from build123d import *

# Parameters (mm, degrees)
PAD_DEPTH       = 3.2
PAD001_DEPTH    = 15.2
POCKET_DEPTH    = 16.6
SKETCH003_R     = 4.1
SKETCH003_R_2   = 1
SKETCH003_R_3   = 3.2
POCKET001_DEPTH = 1.8
SKETCH004_W     = 26.8
SKETCH004_H     = 1.6
PAD002_DEPTH    = 5
CHAMFER_SIZE    = 1.2
POCKET002_DEPTH = 1
SKETCH006_R     = 4.5
SKETCH006_R_2   = 1.7
PAD003_DEPTH    = 3.4
CHAMFER001_SIZE = 0.4
SKETCH007_R     = 1.7
POCKET003_DEPTH = 21.801
SKETCH008_R     = 2.7
POCKET004_DEPTH = 0.6
CHAMFER002_SIZE = 0.8
SKETCH009_R     = 4
POCKET005_DEPTH = 1
SKETCH010_R     = 3
SKETCH010_R_2   = 1.2
PAD004_DEPTH    = 1.6
CHAMFER003_SIZE = 0.4
CHAMFER004_SIZE = 0.8


with BuildPart() as part:
    # Sketch → Pad (new body)
    with BuildSketch(Plane.XY):
        with BuildLine():
            Line((-21, 45), (21, 45))
            ThreePointArc((25, 41), (23.828427, 43.828427), (21, 45))
            Line((25, 41), (25, -41))
            ThreePointArc((21, -45), (23.828427, -43.828427), (25, -41))
            Line((21, -45), (-21, -45))
            ThreePointArc((-25, -41), (-23.828427, -43.828427), (-21, -45))
            Line((-25, -41), (-25, 41))
            ThreePointArc((-21, 45), (-23.828427, 43.828427), (-25, 41))
        make_face()
    extrude(amount=PAD_DEPTH)

    # Sketch001 (on Face9 of Pad) → Pad001 (join)
    with BuildSketch(Plane(origin=(0, 0, 0), x_dir=(1, 0, 0), z_dir=(0, 0, -1))):
        with BuildLine():
            Line((-12, 35), (12, 35))
            ThreePointArc((15, 32), (14.12132, 34.12132), (12, 35))
            Line((15, 32), (15, -32))
            ThreePointArc((12, -35), (14.12132, -34.12132), (15, -32))
            Line((12, -35), (-12, -35))
            ThreePointArc((-15, -32), (-14.12132, -34.12132), (-12, -35))
            Line((-15, -32), (-15, 32))
            ThreePointArc((-12, 35), (-14.12132, 34.12132), (-15, 32))
        make_face()
    extrude(amount=PAD001_DEPTH)

    # Sketch002 (on Face5 of Pad001) → Pocket (cut)
    with BuildSketch(Plane.XY.offset(3.2)):
        with BuildLine():
            Line((-11.2, 33.4), (11.2, 33.4))
            ThreePointArc((13.4, 31.2), (12.755635, 32.755635), (11.2, 33.4))
            Line((13.4, 31.2), (13.4, -31.2))
            ThreePointArc((11.2, -33.4), (12.755635, -32.755635), (13.4, -31.2))
            Line((11.2, -33.4), (-11.2, -33.4))
            ThreePointArc((-13.4, -31.2), (-12.755635, -32.755635), (-11.2, -33.4))
            Line((-13.4, -31.2), (-13.4, 31.2))
            ThreePointArc((-11.2, 33.4), (-12.755635, 32.755635), (-13.4, 31.2))
        make_face()
    extrude(amount=-POCKET_DEPTH, mode=Mode.SUBTRACT)

    # Sketch003 (on Face28 of Pocket) → Pocket001 (cut)
    with BuildSketch(Plane.XY.offset(-13.4)):
        with Locations((0, -24)):
            Circle(SKETCH003_R)
        with Locations((0, -10)):
            Circle(SKETCH003_R_2)
        with Locations((0, 10)):
            Circle(SKETCH003_R_3)
        with Locations((0, 25)):
            Circle(SKETCH003_R_2)
    extrude(amount=-POCKET001_DEPTH, mode=Mode.SUBTRACT)

    # Sketch004 (on Face28 of Pocket001) → Pad002 (join)
    with BuildSketch(Plane.XY.offset(-13.4)):
        Rectangle(SKETCH004_W, SKETCH004_H)
    extrude(amount=PAD002_DEPTH)

    # Chamfer
    chamfer_edges = [part.edges().sort_by_distance(p)[0] for p in [
        (-23.828427, 43.828427, 3.2),
        (-25, 0, 3.2),
        (0, 45, 3.2),
        (23.828427, 43.828427, 3.2),
        (25, 0, 3.2),
        (-23.828427, -43.828427, 3.2),
        (0, -45, 3.2),
        (23.828427, -43.828427, 3.2),
    ]]
    chamfer(chamfer_edges, length=CHAMFER_SIZE)

    # Sketch005 (on Face35 of Chamfer) → Pocket002 (cut)
    with BuildSketch(Plane(origin=(0, 0, -15.2), x_dir=(1, 0, 0), z_dir=(0, 0, -1))):
        with BuildLine():
            ThreePointArc((0.6, -17.1), (1.3, -16.4), (0.6, -15.7))
            Line((0.6, -15.7), (-0.6, -15.7))
            ThreePointArc((-0.6, -15.7), (-1.3, -16.4), (-0.6, -17.1))
            Line((-0.6, -17.1), (0.6, -17.1))
        make_face()
    extrude(amount=-POCKET002_DEPTH, mode=Mode.SUBTRACT)

    # Sketch006 (on Face35 of Pocket002) → Pad003 (join)
    with BuildSketch(Plane(origin=(0, 0, -15.2), x_dir=(1, 0, 0), z_dir=(0, 0, -1))):
        with Locations((0, 10)):
            Circle(SKETCH006_R)
        with Locations((0, 10)):
            Circle(SKETCH006_R_2, mode=Mode.SUBTRACT)
        with Locations((0, -25)):
            Circle(SKETCH006_R)
        with Locations((0, -25)):
            Circle(SKETCH006_R_2, mode=Mode.SUBTRACT)
    extrude(amount=PAD003_DEPTH)

    # Chamfer001
    chamfer001_edges = [part.edges().sort_by_distance(p)[0] for p in [
        (-1, 25, -15.2),
        (-1, -10, -15.2),
    ]]
    chamfer(chamfer001_edges, length=CHAMFER001_SIZE)

    # Sketch007 (on Face13 of Chamfer001) → Pocket003 (cut, through all)
    with BuildSketch(Plane.XY.offset(3.2)):
        with Locations((-19, 39)):
            Circle(SKETCH007_R)
        with Locations((19, 39)):
            Circle(SKETCH007_R)
        with Locations((-19, -39)):
            Circle(SKETCH007_R)
        with Locations((19, -39)):
            Circle(SKETCH007_R)
    extrude(amount=-POCKET003_DEPTH, mode=Mode.SUBTRACT)

    # Sketch008 (on Face13 of Pocket003) → Pocket004 (cut)
    with BuildSketch(Plane.XY.offset(3.2)):
        with Locations((-19, 39)):
            Circle(SKETCH008_R)
        with Locations((19, 39)):
            Circle(SKETCH008_R)
        with Locations((-19, -39)):
            Circle(SKETCH008_R)
        with Locations((19, -39)):
            Circle(SKETCH008_R)
    extrude(amount=-POCKET004_DEPTH, mode=Mode.SUBTRACT)

    # Chamfer002
    chamfer002_edges = [part.edges().sort_by_distance(p)[0] for p in [
        (-20.7, 39, 2.6),
        (17.3, 39, 2.6),
        (17.3, -39, 2.6),
        (-20.7, -39, 2.6),
    ]]
    chamfer(chamfer002_edges, length=CHAMFER002_SIZE)

    # Sketch009 (on Face6 of Chamfer002) → Pocket005 (cut)
    with BuildSketch(Plane(origin=(0, 0, 0), x_dir=(1, 0, 0), z_dir=(0, 0, -1))):
        with Locations((-19, 39)):
            Circle(SKETCH009_R)
        with Locations((19, 39)):
            Circle(SKETCH009_R)
        with Locations((-19, -39)):
            Circle(SKETCH009_R)
        with Locations((19, -39)):
            Circle(SKETCH009_R)
    extrude(amount=-POCKET005_DEPTH, mode=Mode.SUBTRACT)

    # Sketch010 (on Face38 of Pocket005) → Pad004 (join)
    with BuildSketch(Plane.XY.offset(-13.4)):
        with Locations((0, 25)):
            Circle(SKETCH010_R)
        with Locations((0, 25)):
            Circle(SKETCH010_R_2, mode=Mode.SUBTRACT)
        with Locations((0, -10)):
            Circle(SKETCH010_R)
        with Locations((0, -10)):
            Circle(SKETCH010_R_2, mode=Mode.SUBTRACT)
    extrude(amount=PAD004_DEPTH)

    # Chamfer003
    chamfer003_edges = [part.edges().sort_by_distance(p)[0] for p in [
        (-3, 25, -11.8),
        (-3, -10, -11.8),
    ]]
    chamfer(chamfer003_edges, length=CHAMFER003_SIZE)

    # Chamfer004
    chamfer004_edges = [part.edges().sort_by_distance(p)[0] for p in [
        (-1.2, 25, -11.8),
        (-1.2, -10, -11.8),
    ]]
    chamfer(chamfer004_edges, length=CHAMFER004_SIZE)


solid = part.part
Could you check a few things on this model? Use its own coordinates, in mm. A direction names the side the tool comes from. Give positions to 0.01 mm unless a question says otherwise; leave off trailing zeros. Order: outer loops, then holes, each group sorted by start corner. A loop starts at its lowest first (then second) coordinate and runs counter-clockwise, first axis right, second up. Notation, with made-up numbers: (-18, -33.5) -> (7, -33.5) arc R32 ccw to (7, 3.5) -> close; hole circle Ø4 at (-11.5, 64.5). An arc over 180 degrees is marked (long way). Answer in a Markdown table with one row per item. Add a question column.
Item 1: Imagine slicing it at D-D (y = 10). List the corners of the cut face in (x, z) for me.
Item 2: Imagine slicing it at A-A (y = 39). Count the separate pieces of the cut face and the enclosed holes in it, and give its area (3 significant figures).
Item 3: For faces 1 (the flat face through (0, -33.4, -5)), 2 (the flat face through (-25, -1, 1)), 3 (the cylindrical face through (-14.1, -34.14, -7.49)), which set-ups out of +Z, -Z, +X, -X, +Y, -Y let a thin tool reach every point of the face, with its end or its side?
Item 4: I'm going to push flat-ended pins straight in: P1, Ø8, axis at x = -17.5, y = -17, coming from the -Z side; P2, Ø6, axis at x = 12.5, z = -16, coming from the -Y side; P3, Ø1, axis at y = 33, z = -9, coming from the -X side. Where does each tip first touch, or does it pass through?
Item 5: Imagine slicing it at C-C (y = -24). List the corners of the cut face in (x, z) for me.
Item 6: We'd pull the mould along X, two halves only. Please class faces 4 (the cylindrical face through (-0.59, -14.46, -16.88)), 5 (the cylindrical face through (-14.14, 34.1, -7.49)), 6 (the cylindrical face through (-0.221, 23.314, -16.876)): pulls with the +X half, pulls with the -X half, needs draft (parallel to the pull), parting line crosses it, or undercut.
Item 7: Please list where these lines run through material, in increasing order: probe 1 along Y at (x, z) = (19, 1.2); probe 2 along Y at (x, z) = (0, -16); probe 3 along Y at (x, z) = (4, -12.75).
Result:
| question | item | result |
|---|---|---|
| 1 | outline | (-25, 0) -> (-15, 0) -> (-15, -15.2) -> (-3.2, -15.2) -> (-3.2, -13.4) -> (-13.4, -13.4) -> (-13.4, 3.2) -> (-23.8, 3.2) -> (-25, 2) -> close; (3.2, -15.2) -> (15, -15.2) -> (15, 0) -> (25, 0) -> (25, 2) -> (23.8, 3.2) -> (13.4, 3.2) -> (13.4, -13.4) -> (3.2, -13.4) -> close |
| 2 | separate pieces | 3 |
| 2 | enclosed holes | 0 |
| 2 | area | 124 mm2 |
| 3 | face 1 | +Z |
| 3 | face 2 | +Z, -Z, -X, +Y, -Y |
| 3 | face 3 | -Z, -X, -Y |
| 4 | P1 | z = -15.2 |
| 4 | P2 | y = -35 |
| 4 | P3 | x = -14.96 |
| 5 | outline | (-25, 0) -> (-15, 0) -> (-15, -15.2) -> (-4.1, -15.2) -> (-4.1, -13.4) -> (-13.4, -13.4) -> (-13.4, 3.2) -> (-23.8, 3.2) -> (-25, 2) -> close; (4.1, -15.2) -> (15, -15.2) -> (15, 0) -> (25, 0) -> (25, 2) -> (23.8, 3.2) -> (13.4, 3.2) -> (13.4, -13.4) -> (4.1, -13.4) -> close |
| 6 | face 4 | parting line crosses it |
| 6 | face 5 | pulls with the -X half |
| 6 | face 6 | undercut |
| 7 | probe 1 | -45 to -40.7, -37.3 to 37.3, 40.7 to 45 |
| 7 | probe 2 | -14.5 to -11.7, -8.3 to -5.5, 20.5 to 23.3, 26.7 to 29.5 |
| 7 | probe 3 | -35 to -33.4, -0.8 to 0.8, 33.4 to 35 |
